Autodesk Inventor part; units mm, degrees
ref_plane "YZ Plane" through (0, 0, 0) normal (1, 0, 0) x (0, 1, 0)
ref_plane "XZ Plane" through (0, 0, 0) normal (0, 1, 0) x (-1, 0, 0)
ref_plane "XY Plane" through (0, 0, 0) normal (0, 0, 1) x (1, 0, 0)
sketch "Boceto1" plane through (0, 0, 0) normal (0, 1, 0) x (-1, 0, 0)
  arc A0 (20.01, -12.2) -> (20.01, 12.2) centre (24.5, 0) ccw
  arc A1 (-21.2615, 11.0346) -> (-21.2615, -11.0346) centre (-24.5, 0) ccw
  line L0 (-2.1651, 3.75) -> (2.1651, 3.75)
  line L1 (2.1651, 3.75) -> (4.3301, 0)
  line L2 (4.3301, 0) -> (2.1651, -3.75)
  line L3 (2.1651, -3.75) -> (-2.1651, -3.75)
  line L4 (-2.1651, -3.75) -> (-4.3301, 0)
  line L5 (-4.3301, 0) -> (-2.1651, 3.75)
  line L6 (0, 0) -> (0, 8.5) construction
  line L7 (0, 0) -> (0, -8.5) construction
  line L8 (0, 0) -> (2.6275, 0) construction
  arc A2 (20.01, -12.2) -> (-21.4933, -11.1) centre (-2.4996, -77.9761) ccw
  arc A3 (-21.4933, 11.1) -> (20.01, 12.2) centre (-2.4996, 77.9761) ccw
  arc A4 (20.01, 12.2) -> (20.01, -12.2) centre (24.5, 0) ccw construction
  arc A5 (-21.2615, -11.0346) -> (-21.2615, 11.0346) centre (-24.5, 0) ccw construction
  point P0 (-21.4933, 11.1)
  dimension "d2" = 7.5
  dimension "d3" = 49
  dimension "d4" = 8.5
  dimension "d5" = 8.5
  dimension "d6" = 26
  dimension "d7" = 23
  dimension "d12" = 12.2
  dimension "d13" = 11.1
extrude "Extrusión1" add sketch "Boceto1" along normal blind 9
sketch "Boceto2" plane through (0, 9, 0) normal (0, 1, 0) x (1, 0, 0)
  arc A0 (-20.01, 12.2) -> (-20.01, -12.2) centre (-24.5, 0) ccw
  arc A1 (21.4933, -11.1) -> (21.4933, 11.1) centre (24.5, 0) ccw
  arc A2 (-24.5, 6.25) -> (-24.5, -6.25) centre (-24.5, 0) ccw
  arc A3 (24.5, -5.75) -> (24.5, 5.75) centre (24.5, 0) ccw
  arc A4 (-21.3915, 8.4462) -> (-21.3915, -8.4462) centre (-24.5, 0) ccw
  arc A5 (22.5391, -7.2391) -> (22.5391, 7.2391) centre (24.5, 0) ccw
  line L0 (-21.3915, 8.4462) -> (-24.5, 6.25)
  line L1 (-21.3915, -8.4462) -> (-24.5, -6.25)
  arc A6 (-24.5, -6.25) -> (-24.5, 6.25) centre (-24.5, 0) ccw construction
  line L2 (22.5391, 7.2391) -> (24.5, 5.75)
  line L3 (22.5391, -7.2391) -> (24.5, -5.75)
  arc A7 (24.5, 5.75) -> (24.5, -5.75) centre (24.5, 0) ccw construction
  point P0 (0, 0)
  dimension "d16" = 12.5
  dimension "d17" = 11.5
  dimension "d18" = 4
  dimension "d19" = 4
extrude "Extrusión2" cut sketch "Boceto2" against normal up to surface (9 mm away)
sketch "Boceto3" plane through (0, 9, 0) normal (0, 1, 0) x (1, 0, 0)
  arc A0 (-24.5, 6.25) -> (-24.5, -6.25) centre (-24.5, 0) ccw
  arc A1 (24.5, -5.75) -> (24.5, 5.75) centre (24.5, 0) ccw
  arc A2 (-24.2158, 3.3881) -> (-24.2158, -3.3881) centre (-24.5, 0) ccw
  arc A3 (-8.1786, -2.0428) -> (-8.1786, 2.0428) centre (-8.35, 0) ccw
  line L0 (-27.9, 3.184) -> (-27.9, -2.3152) construction
  line L1 (-6.3, 2.5123) -> (-6.3, -1.5596) construction
  line L2 (0, 0) -> (0, -2.3152) construction
  line L3 (-24.2158, 3.3881) -> (-8.1786, 2.0428)
  line L4 (-24.2158, -3.3881) -> (-8.1786, -2.0428)
  arc A4 (24.2158, -3.3881) -> (24.2158, 3.3881) centre (24.5, 0) ccw
  arc A5 (8.1786, 2.0428) -> (8.1786, -2.0428) centre (8.35, 0) ccw
  line L5 (24.2158, 3.3881) -> (8.1786, 2.0428)
  line L6 (24.2158, -3.3881) -> (8.1786, -2.0428)
  arc A6 (-24.2158, -3.3881) -> (-24.2158, 3.3881) centre (-24.5, 0) ccw construction
  arc A7 (-8.1786, 2.0428) -> (-8.1786, -2.0428) centre (-8.35, 0) ccw construction
  arc A8 (8.1786, -2.0428) -> (8.1786, 2.0428) centre (8.35, 0) ccw construction
  arc A9 (24.2158, 3.3881) -> (24.2158, -3.3881) centre (24.5, 0) ccw construction
  dimension "d22" = 6.8
  dimension "d28" = 4.1
  dimension "d30" = 21.6
extrude "Extrusión3" cut sketch "Boceto3" against normal blind 2.5
sketch "Boceto4" plane through (0, 6.5, 0) normal (0, 1, 0) x (1, 0, 0)
  arc A0 (-24.2158, 3.3881) -> (-24.2158, -3.3881) centre (-24.5, 0) ccw
  line L0 (0, 0) -> (0, -3.3881) construction
  arc A1 (-24.2158, 3.3881) -> (-24.2158, -3.3881) centre (-24.5, 0) ccw
  circle A2 centre (-24.5, 0) radius 3.4
  circle A3 centre (-12.3, 0) radius 1
  circle A4 centre (24.5, 0) radius 3.4
  circle A5 centre (12.3, 0) radius 1
  point P0 (-24.2158, -3.3881)
  dimension "d33" = 6.8
  dimension "d34" = 2
  dimension "d35" = 12.2
extrude "Extrusión4" cut sketch "Boceto4" against normal up to surface (6.5 mm away)
sketch "Boceto5" plane through (0, 0, 0) normal (0, -1, 0) x (1, 0, 0)
  circle A0 centre (24.5, 0) radius 3.4
  circle A1 centre (-24.5, 0) radius 3.4
  circle A2 centre (24.5, 0) radius 9.9
  circle A3 centre (-24.5, 0) radius 10.5
  point P0 (0, 0)
  dimension "d38" = 19.8
  dimension "d39" = 21
extrude "Extrusión5" cut sketch "Boceto5" against normal blind 4.1 contours A0 | A1 | A2 | A3
sketch "Boceto6" plane through (0, 0, 0) normal (0, 0, 1) x (1, 0, 0)
  line L0 (-20.01, 9) -> (21.4933, 9)
  line L1 (2.1651, 9) -> (-2.1651, 9)
  line L2 (0, 9) -> (0, 11.4954) construction
  line L3 (-37.5, 0) -> (-37.5, 9)
  line L4 (36, 0) -> (36, 9)
  line L5 (36, 0) -> (21.4933, 0)
  line L6 (-20.01, 0) -> (-37.5, 0)
  arc A0 (27, 0) -> (-28.5, 0) centre (-0.75, -126.8438) ccw
  line L7 (-9.6072, 3) -> (8.7031, 3) construction
  line L8 (-28.5, 0) -> (27, 0)
  line L9 (-20.01, 0) -> (21.4933, 0)
  point P0 (0, 0)
  dimension "d42" = 9
  dimension "d43" = 9
  dimension "d44" = 6
extrude "Extrusión6" cut sketch "Boceto6" along normal through all both and the other way through all
chamfer "Chaflán1" distance 2.5 angle 45 4 edges at (0.6576, 9, -8.4795) (-37.5, 9, 0) (0.6576, 9, 8.4795) (36, 9, 0)
properties part number "Femur_V2"
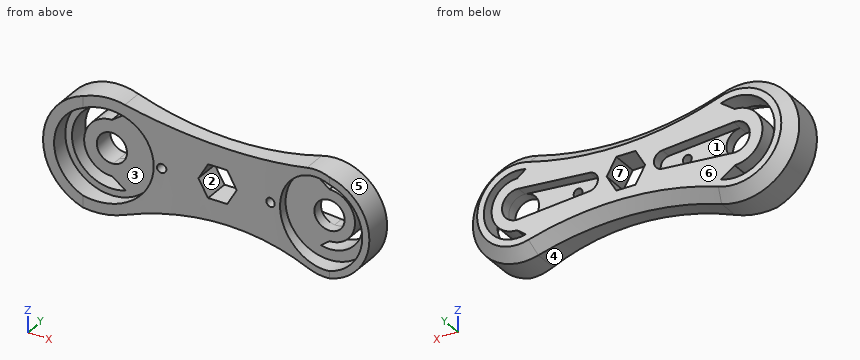
Geometry: final body of the model. Coordinates: model frame, mm. Face numbers are marked on the shaded views. A direction names the side the tool comes from. Round coordinates to 2 decimals unless told otherwise and drop trailing zeros. Loops run counter-clockwise (first coordinate to the right, second up) from the corner with the lowest first, then second, coordinate; pieces in that order, holes last.
Q1. Section A-A on y = 5. Return loops of the section in (x, z).
Q2. Access query for the marked faces 1, 2 and 3. Directions: +Z, -Z, +X, -X, +Y, -Y. A direction counts if a zero-diameter tool reaches every point of the face in a straight line with its end or side. Return the directions, or none.
Q3. Material intervals for L1, parallel to Z at x = 24.5, y = 5.25; L2, parallel to X at y = 5, z = 4.5; L3, parallel to X at y = 8.5, z = 4.25, sorted ascending.
Q4. Pin query (flat end, axial travel): P1, Ø2, axis at x = 12.5, z = -1.5, coming from the +Y side; P2, Ø2, axis at x = 24.5, y = 2, coming from the +Z side; P3, Ø2, axis at x = -16, z = 1.5, coming from the +Y side; P4, Ø6, axis at x = 26.5, z = -2.5, coming from the -Y side. Return the tip coordinate at first contact, or that it passes through.
Q5. Pull-direction query (Z, two-part tool) for the marked faces 4, 5, 6 and 7; classes: released by +Z, released by -Z, zero draft, split by the parting line, or undercut.
Evaluation:
1. outline: (-20.01, -12.2) arc R69.52 cw to (21.26, -11.03) arc R11.5 ccw (long way) to (21.26, 11.03) arc R69.52 cw to (-20.01, 12.2) arc R13 ccw (long way) to start; hole circle Ø6.8 at (-24.5, 0); hole (-24.5, -6.25) arc R6.25 cw to (-24.5, 6.25) - (-21.39, 8.45) arc R9 ccw (long way) to (-21.39, -8.45) - close; hole circle Ø2 at (-12.3, 0); hole (-4.33, 0) - (-2.17, -3.75) - (2.17, -3.75) - (4.33, 0) - (2.17, 3.75) - (-2.17, 3.75) - close; hole circle Ø2 at (12.3, 0); hole circle Ø6.8 at (24.5, 0); hole (22.54, -7.24) arc R7.5 ccw (long way) to (22.54, 7.24) - (24.5, 5.75) arc R5.75 cw to (24.5, -5.75) - close
2. face 1: +Y
2. face 2: +Y, -Y
2. face 3: -Y
3. L1: z = -11.5 to -7.5, -5.75 to -3.4, 3.4 to 5.75, 7.5 to 11.5
3. L2: x = -36.7 to -32.29, -28.84 to 28.08, 30.5 to 35.08
3. L3: x = -34.65 to -32.43, -29.08 to 28.37, 30.68 to 33
4. P1: stops at y = 9
4. P2: stops at z = 11.5
4. P3: stops at y = 6.5
4. P4: stops at y = 4.1
5. face 4: released by -Z
5. face 5: split by the parting line
5. face 6: zero draft
5. face 7: undercut
